```python
from build123d import *

# Parameters (mm, degrees)
SKETCH_1_R          = 13.5
SKETCH_1_R_2        = 1.5
SKETCH_1_R_3        = 1.3
EXTRUDE_1_DEPTH     = 4
SKETCH_2_W          = 19
SKETCH_2_H          = 13
SKETCH_2_W_2        = 9.5
SKETCH_2_H_2        = 35
SKETCH_2_H_3        = 25
CUT_EXTRUDE_1_DEPTH = 152.091561644
FILLET_1_R          = 2.5


with BuildPart() as part:
    # 草图1 → 凸台-拉伸1 (new body)
    with BuildSketch(Plane(origin=(0, 0, 0), x_dir=(1, 0, 0), z_dir=(0, 1, 0))):
        with BuildLine():
            Line((16.5, 103.5), (-16.5, 103.5))
            Line((-16.5, 103.5), (-16.5, 90.5))
            Line((-16.5, 90.5), (-36.9, 90.5))
            ThreePointArc((-36.9, 90.5), (-57.866998484, 70.67684942), (-39.25, 48.631902339))
            Line((-39.25, 48.631902339), (-39.25, -39.5))
            Line((-39.25, -39.5), (-39.25, -139.5))
            Line((-39.25, -139.5), (23.75, -139.5))
            Line((23.75, -139.5), (23.75, -39.5))
            Line((23.75, -39.5), (23.75, -34.5))
            Line((23.75, -34.5), (23.75, 34.5))
            Line((23.75, 34.5), (23.75, 48.5))
            Line((23.75, 48.5), (36.9, 48.5))
            ThreePointArc((36.9, 48.5), (57.9, 69.5), (36.9, 90.5))
            Line((36.9, 90.5), (16.5, 90.5))
            Line((16.5, 90.5), (16.5, 103.5))
        make_face()
        with Locations(Location((-36.9, 69.5, 0), (0, 0, 270))):
            Circle(SKETCH_1_R, mode=Mode.SUBTRACT)
        with Locations(Location((-36.9, 87, 0), (0, 0, 270))):
            Circle(SKETCH_1_R_2, mode=Mode.SUBTRACT)
        with Locations(Location((-24.525631329, 81.874368671, 0), (0, 0, 270))):
            Circle(SKETCH_1_R_2, mode=Mode.SUBTRACT)
        with Locations(Location((-19.4, 69.5, 0), (0, 0, 270))):
            Circle(SKETCH_1_R_2, mode=Mode.SUBTRACT)
        with Locations(Location((-24.525631329, 57.125631329, 0), (0, 0, 270))):
            Circle(SKETCH_1_R_2, mode=Mode.SUBTRACT)
        with Locations(Location((-36.9, 52, 0), (0, 0, 270))):
            Circle(SKETCH_1_R_2, mode=Mode.SUBTRACT)
        with Locations(Location((-49.274368671, 57.125631329, 0), (0, 0, 270))):
            Circle(SKETCH_1_R_2, mode=Mode.SUBTRACT)
        with Locations(Location((-54.4, 69.5, 0), (0, 0, 270))):
            Circle(SKETCH_1_R_2, mode=Mode.SUBTRACT)
        with Locations(Location((-49.274368671, 81.874368671, 0), (0, 0, 270))):
            Circle(SKETCH_1_R_2, mode=Mode.SUBTRACT)
        with Locations(Location((-13, 99.5, 0), (0, 0, 270))):
            Circle(SKETCH_1_R_2, mode=Mode.SUBTRACT)
        with Locations(Location((-13, 39.5, 0), (0, 0, 270))):
            Circle(SKETCH_1_R_2, mode=Mode.SUBTRACT)
        with Locations(Location((13, 39.5, 0), (0, 0, 90))):
            Circle(SKETCH_1_R_2, mode=Mode.SUBTRACT)
        with Locations(Location((13, 99.5, 0), (0, 0, 90))):
            Circle(SKETCH_1_R_2, mode=Mode.SUBTRACT)
        with Locations(Location((54.4, 69.5, 0), (0, 0, 90))):
            Circle(SKETCH_1_R_2, mode=Mode.SUBTRACT)
        with Locations(Location((49.274368671, 57.125631329, 0), (0, 0, 90))):
            Circle(SKETCH_1_R_2, mode=Mode.SUBTRACT)
        with Locations(Location((36.9, 52, 0), (0, 0, 90))):
            Circle(SKETCH_1_R_2, mode=Mode.SUBTRACT)
        with Locations(Location((24.525631329, 57.125631329, 0), (0, 0, 90))):
            Circle(SKETCH_1_R_2, mode=Mode.SUBTRACT)
        with Locations(Location((19.4, 69.5, 0), (0, 0, 90))):
            Circle(SKETCH_1_R_2, mode=Mode.SUBTRACT)
        with Locations(Location((24.525631329, 81.874368671, 0), (0, 0, 90))):
            Circle(SKETCH_1_R_2, mode=Mode.SUBTRACT)
        with Locations(Location((36.9, 87, 0), (0, 0, 90))):
            Circle(SKETCH_1_R_2, mode=Mode.SUBTRACT)
        with Locations(Location((49.274368671, 81.874368671, 0), (0, 0, 90))):
            Circle(SKETCH_1_R_2, mode=Mode.SUBTRACT)
        with Locations(Location((36.9, 69.5, 0), (0, 0, 90))):
            Circle(SKETCH_1_R, mode=Mode.SUBTRACT)
        with Locations(Location((-13, 29.5, 0), (0, 0, 270))):
            Circle(SKETCH_1_R_2, mode=Mode.SUBTRACT)
        with Locations(Location((-35.75, -42.5, 0), (0, 0, 270))):
            Circle(SKETCH_1_R_2, mode=Mode.SUBTRACT)
        with Locations(Location((-35.75, -136.5, 0), (0, 0, 90))):
            Circle(SKETCH_1_R_2, mode=Mode.SUBTRACT)
        with Locations(Location((20.25, -136.5, 0), (0, 0, 270))):
            Circle(SKETCH_1_R_2, mode=Mode.SUBTRACT)
        with Locations(Location((20.25, -42.5, 0), (0, 0, 90))):
            Circle(SKETCH_1_R_2, mode=Mode.SUBTRACT)
        with Locations(Location((13, 29.5, 0), (0, 0, 90))):
            Circle(SKETCH_1_R_2, mode=Mode.SUBTRACT)
        with Locations(Location((20.75, 15, 0), (0, 0, 270))):
            Circle(SKETCH_1_R_2, mode=Mode.SUBTRACT)
        with Locations(Location((20.75, -15, 0), (0, 0, 90))):
            Circle(SKETCH_1_R_2, mode=Mode.SUBTRACT)
        with Locations(Location((-28.75, -58, 0), (0, 0, 270))):
            Circle(SKETCH_1_R_3, mode=Mode.SUBTRACT)
        with Locations(Location((-28.75, -121, 0), (0, 0, 90))):
            Circle(SKETCH_1_R_3, mode=Mode.SUBTRACT)
        with Locations(Location((13.25, -121, 0), (0, 0, 270))):
            Circle(SKETCH_1_R_3, mode=Mode.SUBTRACT)
        with Locations(Location((13.25, -58, 0), (0, 0, 90))):
            Circle(SKETCH_1_R_3, mode=Mode.SUBTRACT)
        with Locations(Location((-9.25, -20, 0), (0, 0, 270))):
            Circle(SKETCH_1_R_2, mode=Mode.SUBTRACT)
        with Locations(Location((20.75, 39.5, 0), (0, 0, 270))):
            Circle(SKETCH_1_R_2, mode=Mode.SUBTRACT)
        with Locations(Location((-20.75, 39.5, 0), (0, 0, 90))):
            Circle(SKETCH_1_R_2, mode=Mode.SUBTRACT)
        with Locations(Location((20.75, 29.5, 0), (0, 0, 90))):
            Circle(SKETCH_1_R_2, mode=Mode.SUBTRACT)
        with Locations(Location((-20.75, 29.5, 0), (0, 0, 270))):
            Circle(SKETCH_1_R_2, mode=Mode.SUBTRACT)
        with Locations(Location((20.75, -30.5, 0), (0, 0, 90))):
            Circle(SKETCH_1_R_2, mode=Mode.SUBTRACT)
        with Locations(Location((-20.75, -30.5, 0), (0, 0, 270))):
            Circle(SKETCH_1_R_2, mode=Mode.SUBTRACT)
    extrude(amount=EXTRUDE_1_DEPTH)

    # 草图2 → 切除-拉伸1 (cut, through all)
    with BuildSketch(Plane(origin=(0, 4, 0), x_dir=(1, 0, 0), z_dir=(0, 1, 0))):
        with Locations((0, 97)):
            Rectangle(SKETCH_2_W, SKETCH_2_H)
        Polygon((-33.25, -45.5), (17.75, -45.5), (17.75, -55.5), (10.75, -55.5), (10.75, -60.5), (17.75, -60.5), (17.75, -118.5), (10.75, -118.5), (10.75, -123.5), (17.75, -123.5), (17.75, -133.5), (-33.25, -133.5), (-33.25, -123.5), (-26.25, -123.5), (-26.25, -118.5), (-33.25, -118.5), (-33.25, -60.5), (-26.25, -60.5), (-26.25, -55.5), (-33.25, -55.5), align=None)
        with Locations((-28.5, 31.319634916)):
            Rectangle(SKETCH_2_W_2, SKETCH_2_H_2)
        with Locations((-28.5, -13.680365084)):
            Rectangle(SKETCH_2_W_2, SKETCH_2_H_2)
        with Locations((0, 36)):
            Rectangle(SKETCH_2_W, SKETCH_2_H_3)
    extrude(amount=-CUT_EXTRUDE_1_DEPTH, mode=Mode.SUBTRACT)

    # 圆角1
    fillet_1_edges = [part.edges().sort_by_distance(p)[0] for p in [
        (23.75, 2, 139.5),
        (-39.25, 2, 139.5),
        (-33.25, 2, 123.5),
        (-26.25, 2, 123.5),
        (-33.25, 2, 118.5),
        (-26.25, 2, 118.5),
        (-33.25, 2, 133.5),
        (17.75, 2, 133.5),
        (17.75, 2, 123.5),
        (10.75, 2, 123.5),
        (10.75, 2, 118.5),
        (17.75, 2, 118.5),
        (17.75, 2, 55.5),
        (17.75, 2, 60.5),
        (10.75, 2, 60.5),
        (10.75, 2, 55.5),
        (-33.25, 2, 60.5),
        (-26.25, 2, 60.5),
        (-26.25, 2, 55.5),
        (-33.25, 2, 55.5),
        (17.75, 2, 45.5),
        (-33.25, 2, 45.5),
        (-33.25, 2, 31.180365084),
        (-23.75, 2, 31.180365084),
        (-23.75, 2, -13.819634916),
        (-33.25, 2, -13.819634916),
        (-23.75, 2, -3.819634916),
        (-33.25, 2, -3.819634916),
        (-33.25, 2, -48.819634916),
        (-23.75, 2, -48.819634916),
        (-39.25, 2, -48.631902339),
        (-16.5, 2, -90.5),
        (9.5, 2, -90.5),
        (16.5, 2, -90.5),
        (16.5, 2, -103.5),
        (9.5, 2, -103.5),
        (-9.5, 2, -90.5),
        (-9.5, 2, -103.5),
        (-16.5, 2, -103.5),
        (-9.5, 2, -23.5),
        (9.5, 2, -23.5),
        (9.5, 2, -48.5),
        (-9.5, 2, -48.5),
    ]]
    fillet(fillet_1_edges, radius=FILLET_1_R - 0.0001)  # a hair under: the kernel refuses the full size


solid = part.part
```
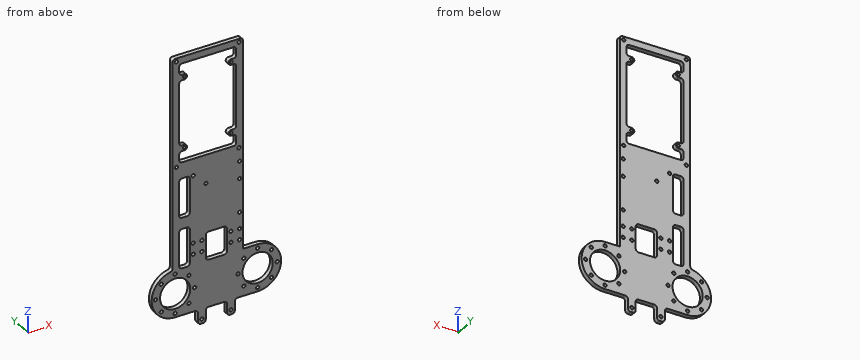
Part model, mm, in its own coordinate system. Give positions to 0.01 mm unless a question says otherwise; leave off trailing zeros. Write each loop counter-clockwise with the first axis right and the second up, starting at its lowest first coordinate (ties: lowest second). Pieces come first, ordered by that corner, then holes. Notation, with made-up numbers: (73, 37.5) -> (123, 37.5) arc R22 ccw to (123, 76.5) -> close; hole circle Ø9 at (0, 17). An arc over 180 degrees is marked (long way). Put each result on its own line as item: value. Start each with the question number.
Item 1: Wall check: L1, parallel to X at y = 2.1, z = 20; L2, parallel to X at y = 2.95, z = 108; L3, parallel to Z at x = 36.9, y = 2.3. Give the ranges that are in metal, low to high. Write a range as [from, to].
Item 2: Pin check, flat tips, straight feed: pin 1 Ø1.6 at (x, z) = (-28.75, 58) entering from +Y (3 decimals); pin 2 Ø1 at (y, z) = (3, 33.5) entering from -X. Stop position of each tip, or through.
Item 3: Cut at B-B (y = 1.75). State how many separate pieces and enclosed holes the cut face has, then the cut area to 3 significant figures.
Item 4: Cut at A-A (x = -45.5). List the corners of the cut face in (y, z), then the cut area to 3 significant figures.
Answer list:
1. L1: x = [-39.25, -33.25], [-23.75, -10.75], [-7.75, 23.75]
1. L2: x = [-39.25, -33.25], [17.75, 23.75]
1. L3: z = [-90.5, -88.5], [-85.5, -83], [-56, -53.5], [-50.5, -48.5]
2. pin 1: passes through
2. pin 2: stops at x = -39.25
3. separate pieces: 1
3. enclosed holes: 45
3. area: 9,630 mm2
4. outline: (0, -88.66) -> (4, -88.66) -> (4, -79.91) -> (0, -79.91) -> close; (0, -59.09) -> (4, -59.09) -> (4, -50.34) -> (0, -50.34) -> close
4. area: 70.0 mm2
